For this review, use the dimensioned drawing (mm, ordinates from the lowest corner) and the shaded views. Round coordinates to 2 decimals unless told otherwise and drop trailing zeros. Write each loop counter-clockwise with the first axis right and the second up, starting at its lowest first coordinate (ties: lowest second). Pieces come first, ordered by that corner, then holes. Notation, with made-up numbers: (52, -37.75) - (69, -37.75) arc R14 ccw to (69, -13.75) - close; hole circle Ø1 at (13, 68). An arc over 180 degrees is marked (long way). Return JSON: item names as keys, results as strings.
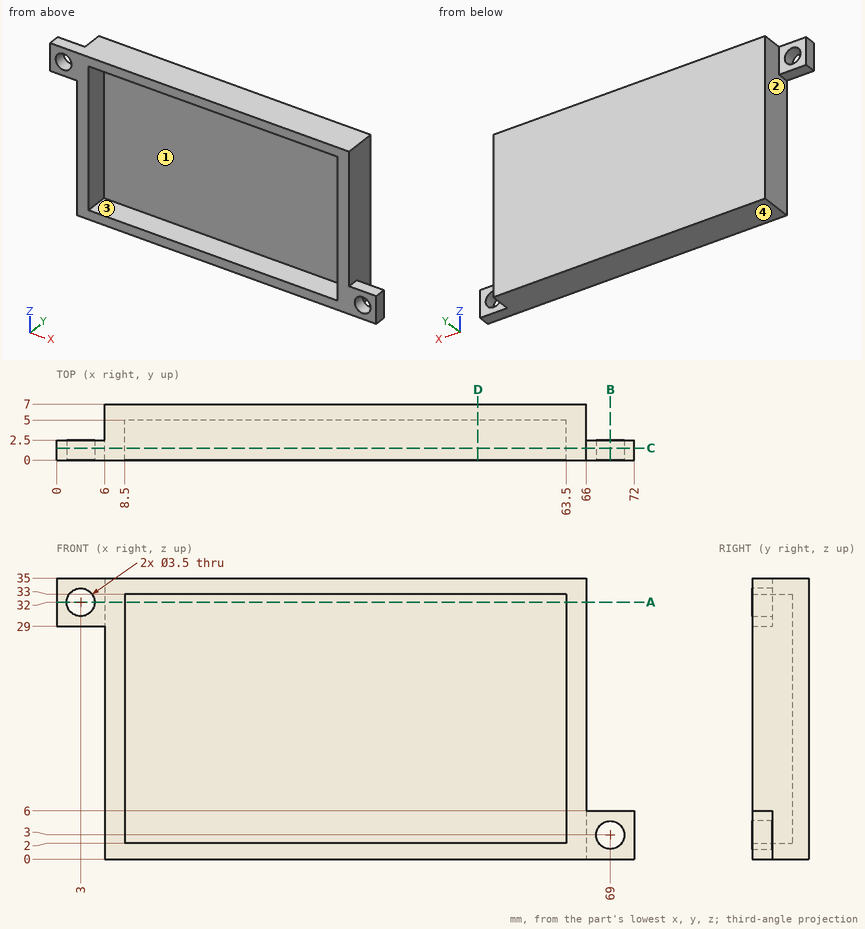
(1) Mouldability with a two-part tool opening along Z and no side actions: class the marked faces 1, 2, 3 and 4 as released by +Z, released by -Z, zero draft, split by the parting line, or undercut.
Filled in:
{"face 1": "undercut", "face 2": "zero draft", "face 3": "undercut", "face 4": "released by -Z"}
(2) Add section D-D (x = 52.5). Write out the cut boundary in (y, z), plus the area to 3 significant figures.
Filled in:
{"outline": "(0, 0) - (7, 0) - (7, 35) - (0, 35) - (0, 33) - (5, 33) - (5, 2) - (0, 2) - close", "area": "90.0 mm2"}
(3) Add section A-A (z = 32). Write out the cut boundary in (x, y), plus the area to 3 significant figures.
Filled in:
{"outline": "(0, 0) - (1.25, 0) - (1.25, 2.5) - (0, 2.5) - close; (4.75, 0) - (8.5, 0) - (8.5, 5) - (63.5, 5) - (63.5, 0) - (66, 0) - (66, 7) - (6, 7) - (6, 2.5) - (4.75, 2.5) - close", "area": "151 mm2"}
(4) Add section C-C (y = 1.5). Write out the cut boundary in (x, z).
Filled in:
{"outline": "(0, 29) - (6, 29) - (6, 0) - (72, 0) - (72, 6) - (66, 6) - (66, 35) - (0, 35) - close; hole circle Ø3.5 at (3, 32); hole (8.5, 2) - (63.5, 2) - (63.5, 33) - (8.5, 33) - close; hole circle Ø3.5 at (69, 3)"}
(5) Add section B-B (x = 69). Write out the cut boundary in (y, z), plus the area to 3 significant figures.
Filled in:
{"outline": "(0, 0) - (2.5, 0) - (2.5, 1.25) - (0, 1.25) - close; (0, 4.75) - (2.5, 4.75) - (2.5, 6) - (0, 6) - close", "area": "6.25 mm2"}
(6) Wall thickness on line 1 (X direction, y = 0.85, z = 32); line 2 (Z direction, x = 44, y = 4); line 3 (Z direction, x = 69, y = 1.15): over which ranges is each line inside the solid? List them lowest first.
Filled in:
{"line 1": "x = 0 to 1.25, 4.75 to 8.5, 63.5 to 66", "line 2": "z = 0 to 2, 33 to 35", "line 3": "z = 0 to 1.25, 4.75 to 6"}
(7) Clearance check with flat-ended pins moving along their axes: pin 1 Ø2.5 at (y, z) = (1.5, 24) entering from +X; pin 2 Ø1 at (y, z) = (0.5, 17) entering from -X; pin 3 Ø5.5 at (x, z) = (69, 3) entering from +Y. State where each tip first meets the part, or that it passes through.
Filled in:
{"pin 1": "stops at x = 66", "pin 2": "stops at x = 6", "pin 3": "stops at y = 2.5"}
